Answer from the drawing. Dimensions are ordinates in mm from the lowest x, y and z of the part. A direction names the side the tool comes from. Round coordinates to 2 decimals unless told otherwise and drop trailing zeros. Loops run counter-clockwise (first coordinate to the right, second up) from the corner with the lowest first, then second, coordinate; pieces in that order, holes last. Notation, with made-up numbers: (57.5, 25) - (78.5, 25) arc R13 cw to (78.5, 37) - close; hole circle Ø2 at (-36, 20.25). An arc over 180 degrees is marked (long way). Answer as CSV lines item,"result".
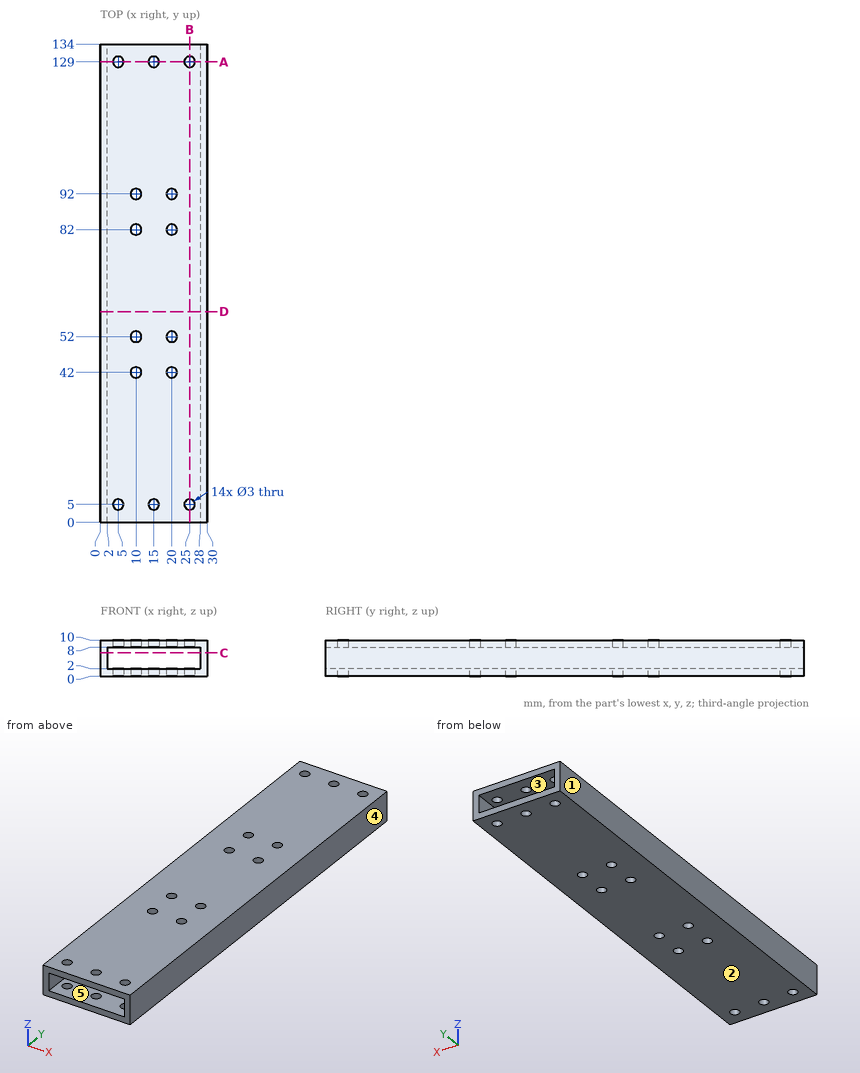
1) A cutting plane is placed at D-D, the plane y = 59. Determine the outline of the cut face in (x, z), plus the area to 3 significant figures.
Entries:
outline,"(0, 0) - (30, 0) - (30, 10) - (0, 10) - close; hole (2, 2) - (28, 2) - (28, 8) - (2, 8) - close"
area,"144 mm^2"
2) This flat-tipped pin is pushed along its axis until it touches: P1, Ø1.8, axis at x = 25, y = 5, coming from the +Z side. Where does it stop, or does it pass through?
Entries:
P1,"passes through"
3) The mould has two halves that part along Z. Classify the marked faces 1, 2 and 3: pulls with the +Z half, pulls with the -Z half, needs draft (parallel to the pull), parting line crosses it, or undercut.
Entries:
face 1,"needs draft"
face 2,"pulls with the -Z half"
face 3,"undercut"
4) A cutting plane is placed at C-C, the plane z = 6.5. Determine the outline of the cut face in (x, y).
Entries:
outline,"(0, 0) - (2, 0) - (2, 134) - (0, 134) - close; (28, 0) - (30, 0) - (30, 134) - (28, 134) - close"
5) Find the intervals of material crossed by line 1 (Y direction, x = 10, z = 1); line 2 (Y direction, x = 25, z = 1.45); line 3 (X direction, y = 92, z = 0.5), in increasing order.
Entries:
line 1,"y = 0 to 40.5, 43.5 to 50.5, 53.5 to 80.5, 83.5 to 90.5, 93.5 to 134"
line 2,"y = 0 to 3.5, 6.5 to 127.5, 130.5 to 134"
line 3,"x = 0 to 8.5, 11.5 to 18.5, 21.5 to 30"
6) A cutting plane is placed at A-A, the plane y = 129. Count the separate pieces of the cut face and the enclosed holes in it, plus the area to 3 significant figures.
Entries:
separate pieces,"6"
enclosed holes,"0"
area,"108 mm^2"
7) A cutting plane is placed at B-B, the plane x = 25. Determine the outline of the cut face in (y, z), plus the area to 3 significant figures.
Entries:
outline,"(0, 0) - (3.5, 0) - (3.5, 2) - (0, 2) - close; (0, 8) - (3.5, 8) - (3.5, 10) - (0, 10) - close; (6.5, 0) - (127.5, 0) - (127.5, 2) - (6.5, 2) - close; (6.5, 8) - (127.5, 8) - (127.5, 10) - (6.5, 10) - close; (130.5, 0) - (134, 0) - (134, 2) - (130.5, 2) - close; (130.5, 8) - (134, 8) - (134, 10) - (130.5, 10) - close"
area,"512 mm^2"
8) A tool of negligible diameter and unlimited length cuts with its end or side. For the marked faces 4 and 5, from which of +Z, -Z, +X, -X, +Y, -Y can it reach the whole face along a straight path? Write none if from no direction.
Entries:
face 4,"+Z, -Z, +X, +Y, -Y"
face 5,"+Y, -Y"
